```python
from build123d import *

# Parameters (mm, degrees)
SKETCH1_W                           = 69.85
SKETCH1_H                           = 53.34
BOSS_EXTRUDE1_DEPTH                 = 3.175
F_1_2_CLEARANCE_HOLE1_D             = 13.09624
F_1_2_CLEARANCE_HOLE1_DEPTH         = 25.4
F_1_2_CLEARANCE_HOLE1_TIP           = 3.934507437
M3_CLEARANCE_HOLE1_D                = 3.2
M3_CLEARANCE_HOLE1_DEPTH            = 25.4
M3_CLEARANCE_HOLE1_TIP              = 0.96137699
F_2_0MM_CLEARANCE_DOWEL_HOLE1_D     = 2
F_2_0MM_CLEARANCE_DOWEL_HOLE1_DEPTH = 25.4
F_2_0MM_CLEARANCE_DOWEL_HOLE1_TIP   = 0.600860619
F_3_0MM_CLEARANCE_DOWEL_HOLE1_D     = 3
F_3_0MM_CLEARANCE_DOWEL_HOLE1_DEPTH = 25.4
F_3_0MM_CLEARANCE_DOWEL_HOLE1_TIP   = 0.901290929
F_5_0MM_CLEARANCE_DOWEL_HOLE1_D     = 5
F_5_0MM_CLEARANCE_DOWEL_HOLE1_DEPTH = 25.4
F_5_0MM_CLEARANCE_DOWEL_HOLE1_TIP   = 1.502151548
CUT_EXTRUDE1_DEPTH                  = 88.94463443
F_4_CLEARANCE_HOLE1_D               = 2.9464
F_4_CLEARANCE_HOLE1_DEPTH           = 3.175
F_4_CLEARANCE_HOLE1_TIP             = 0.885187864


with BuildPart() as part:
    # Sketch1 → Boss-Extrude1 (new body)
    with BuildSketch(Plane(origin=(0, 0, 0), x_dir=(0, 0, -1), z_dir=(1, 0, 0))):
        with Locations((34.925, 26.67)):
            Rectangle(SKETCH1_W, SKETCH1_H)
    extrude(amount=BOSS_EXTRUDE1_DEPTH)

    # 1/2 Clearance Hole1
    with Locations(Plane(origin=(3.175, 0, 0), x_dir=(0, 0, -1), z_dir=(1, 0, 0))):
        with Locations((27.33778886, 21.18693756)):
            Hole(F_1_2_CLEARANCE_HOLE1_D / 2, depth=F_1_2_CLEARANCE_HOLE1_DEPTH)
            with Locations((0, 0, -(F_1_2_CLEARANCE_HOLE1_DEPTH + F_1_2_CLEARANCE_HOLE1_TIP / 2))):  # 118° drill point
                Cone(0, F_1_2_CLEARANCE_HOLE1_D / 2, F_1_2_CLEARANCE_HOLE1_TIP, mode=Mode.SUBTRACT)

    # M3 Clearance Hole1
    with Locations(Plane.ZY):
        with Locations((-40.03778886, 21.18693756), (-33.68778886, 32.185460188), (-20.98778886, 32.185460188), (-14.63778886, 21.18693756), (-20.98778886, 10.188414932), (-33.68778886, 10.188414932), (-27.33778886, 21.18693756)):
            Hole(M3_CLEARANCE_HOLE1_D / 2, depth=M3_CLEARANCE_HOLE1_DEPTH)
            with Locations((0, 0, -(M3_CLEARANCE_HOLE1_DEPTH + M3_CLEARANCE_HOLE1_TIP / 2))):  # 118° drill point
                Cone(0, M3_CLEARANCE_HOLE1_D / 2, M3_CLEARANCE_HOLE1_TIP, mode=Mode.SUBTRACT)

    # Ø2.0mm Clearance Dowel Hole1
    with Locations(Plane(origin=(3.175, 0, 0), x_dir=(0, 0, -1), z_dir=(1, 0, 0))):
        with Locations((37.59058776, 24.95127344)):
            Hole(F_2_0MM_CLEARANCE_DOWEL_HOLE1_D / 2, depth=F_2_0MM_CLEARANCE_DOWEL_HOLE1_DEPTH)
            with Locations((0, 0, -(F_2_0MM_CLEARANCE_DOWEL_HOLE1_DEPTH + F_2_0MM_CLEARANCE_DOWEL_HOLE1_TIP / 2))):  # 118° drill point
                Cone(0, F_2_0MM_CLEARANCE_DOWEL_HOLE1_D / 2, F_2_0MM_CLEARANCE_DOWEL_HOLE1_TIP, mode=Mode.SUBTRACT)

    # Ø3.0mm Clearance Dowel Hole1
    with Locations(Plane(origin=(3.175, 0, 0), x_dir=(0, 0, -1), z_dir=(1, 0, 0))):
        with Locations((51.24750482, 29.46260554)):
            Hole(F_3_0MM_CLEARANCE_DOWEL_HOLE1_D / 2, depth=F_3_0MM_CLEARANCE_DOWEL_HOLE1_DEPTH)
            with Locations((0, 0, -(F_3_0MM_CLEARANCE_DOWEL_HOLE1_DEPTH + F_3_0MM_CLEARANCE_DOWEL_HOLE1_TIP / 2))):  # 118° drill point
                Cone(0, F_3_0MM_CLEARANCE_DOWEL_HOLE1_D / 2, F_3_0MM_CLEARANCE_DOWEL_HOLE1_TIP, mode=Mode.SUBTRACT)

    # Ø5.0mm Clearance Dowel Hole1
    with Locations(Plane(origin=(3.175, 0, 0), x_dir=(0, 0, -1), z_dir=(1, 0, 0))):
        with Locations((56.78027506, 46.53348834)):
            Hole(F_5_0MM_CLEARANCE_DOWEL_HOLE1_D / 2, depth=F_5_0MM_CLEARANCE_DOWEL_HOLE1_DEPTH)
            with Locations((0, 0, -(F_5_0MM_CLEARANCE_DOWEL_HOLE1_DEPTH + F_5_0MM_CLEARANCE_DOWEL_HOLE1_TIP / 2))):  # 118° drill point
                Cone(0, F_5_0MM_CLEARANCE_DOWEL_HOLE1_D / 2, F_5_0MM_CLEARANCE_DOWEL_HOLE1_TIP, mode=Mode.SUBTRACT)

    # Sketch12 → Cut-Extrude1 (cut, through all)
    with BuildSketch(Plane(origin=(3.175, 0, 0), x_dir=(0, 0, -1), z_dir=(1, 0, 0))):
        Polygon((0, 53.34), (50.313533093, 53.34), (0, 26.67), align=None)
        Polygon((69.85, 0), (38.1, 0), (69.85, 33.02), align=None)
        Polygon((25.4, 0), (0, 19.05), (0, 0), align=None)
    extrude(amount=-CUT_EXTRUDE1_DEPTH, mode=Mode.SUBTRACT)

    # #4 Clearance Hole1
    with Locations(Plane(origin=(3.175, 0, 0), x_dir=(0, 0, -1), z_dir=(1, 0, 0))):
        with Locations((3.81, 25.4), (36.83, 3.175), (66.08666234, 32.62292688), (38.1, 39.878)):
            Hole(F_4_CLEARANCE_HOLE1_D / 2, depth=F_4_CLEARANCE_HOLE1_DEPTH)
            with Locations((0, 0, -(F_4_CLEARANCE_HOLE1_DEPTH + F_4_CLEARANCE_HOLE1_TIP / 2))):  # 118° drill point
                Cone(0, F_4_CLEARANCE_HOLE1_D / 2, F_4_CLEARANCE_HOLE1_TIP, mode=Mode.SUBTRACT)


solid = part.part
```
Input: part model. Units: mm. Frame: model coordinates. Coordinates: 2 decimals unless noted, no trailing zeros. Loops run counter-clockwise (first coordinate to the right, second up) from the corner with the lowest first, then second, coordinate; pieces in that order, holes last. Notation, with made-up numbers: (-31.75, 58) -> (4.25, 58) arc R36 ccw to (4.25, 92) -> close; hole circle Ø1 at (9.25, -18.75). An arc over 180 degrees is marked (long way). Use a Markdown table: item, result.
1) Cut plane D-D (z = -3.81). Return the cut outline in (x, y) (1 decimal), then the cut area to 3 significant figures.
Results found:
| item | result |
|---|---|
| outline | (0, 16.2) -> (3.2, 16.2) -> (3.2, 23.9) -> (0, 23.9) -> close; (0, 26.9) -> (3.2, 26.9) -> (3.2, 28.7) -> (0, 28.7) -> close |
| area | 30.3 mm2 |
2) Cut plane A-A (y = 11). Return the cut outline in (x, z) (3 decimals).
Results found:
| item | result |
|---|---|
| outline | (0, -48.677) -> (3.175, -48.677) -> (3.175, -35.067) -> (0, -35.067) -> close; (0, -32.309) -> (3.175, -32.309) -> (3.175, -22.367) -> (0, -22.367) -> close; (0, -19.609) -> (3.175, -19.609) -> (3.175, -10.733) -> (0, -10.733) -> close |
3) Cut plane C-C (x = 2.45). Give the number of separate pieces and of enclosed holes in the cut face, then the cut area to 3 significant figures.
Results found:
| item | result |
|---|---|
| separate pieces | 1 |
| enclosed holes | 14 |
| area | 2,050 mm2 |
4) Contact query for flat-ended pins moving along their axis: pin 1 (1 mm diameter, centred on x = 0.5, z = -48.5, fed in from -Y); pin 2 (1.5 mm diameter, centred on x = 1, y = 32, fed in from -Z). Output: stop coordinate, or through.
Results found:
| item | result |
|---|---|
| pin 1 | stops at y = 10.3 |
| pin 2 | stops at z = -69.59 |
5) Material intervals for line 1 along Y through (x, z) = (1.6, -39); line 2 along Z through (x, y) = (2.6, 21.5); line 3 along Z through (x, y) = (1.45, 9), sorted ascending. Write a range as from..to.
Results found:
| item | result |
|---|---|
| line 1 | y = 0.94..19.97, 22.4..38.71, 41.04..47.34 |
| line 2 | z = -58.77..-41.61, -38.47..-33.88, -20.8..-16.21, -13.07..0 |
| line 3 | z = -46.75..-34.76, -32.62..-22.06, -19.92..-13.4 |
6) Pull-direction query (Z, two-part tool) for faces 1 (the flat face through (2, 43, -69.85)), 2 (the flat face through (2, 53.34, -60)), 3 (the cylindrical face through (1.57, 41.34, -38.29)); classes: released by +Z, released by -Z, zero draft, split by the parting line, or undercut.
Results found:
| item | result |
|---|---|
| face 1 | released by -Z |
| face 2 | zero draft |
| face 3 | undercut |
